Geometry: final body of the model. Coordinates: model frame, mm. Face numbers are marked on the shaded views. Coordinates: 2 decimals unless noted, no trailing zeros. Order: outer loops, then holes, each group sorted by start corner. A loop starts at its lowest first (then second) coordinate and runs counter-clockwise, first axis right, second up. Notation, with made-up numbers: M 65,31 L 116,31 A28 cw 116,51 Z; hole C 77,85 d1. An arc over 180 degrees is marked long. Write item = value, one per line.
from build123d import *

# Parameters (mm, degrees)
SALIENTE_EXTRUIR1_DEPTH = 0.5
CORTAR_EXTRUIR4_REACH   = 2.5
CROQUIS6_R              = 1.585
CORTAR_EXTRUIR5_REACH   = 2.5
CROQUIS7_R              = 1.585
CROQUIS8_R              = 1.585
CORTAR_EXTRUIR6_DEPTH   = 0.5
CROQUIS9_R              = 1.585
CORTAR_EXTRUIR7_DEPTH   = 0.5
CROQUIS5_R              = 1.585
CORTAR_EXTRUIR8_DEPTH   = 0.5
CORTAR_EXTRUIR9_REACH   = 182
CORTAR_EXTRUIR10_START  = -110.74
CORTAR_EXTRUIR10_DEPTH  = 110.74


with BuildPart() as part:
    # Croquis2 → Saliente-Extruir1 (new body)
    with BuildSketch(Plane(origin=(0, 0, 0), x_dir=(1, 0, 0), z_dir=(0, 1, 0))):
        Polygon((-90, 25.54), (-62.5, 25.54), (-62.5, 89.31), (62.5, 89.31), (62.5, 25.54), (90, 25.54), (90, -85.2), (-90, -85.2), align=None)
    saliente_extruir1 = extrude(amount=SALIENTE_EXTRUIR1_DEPTH)

    # Croquis6 → Cortar-Extruir4 (cut, up to next)
    with BuildSketch(Plane(origin=(0, 0.5, 0), x_dir=(1, 0, 0), z_dir=(0, 1, 0)), mode=Mode.PRIVATE) as cortar_extruir4_sk1:
        with Locations((-56.5, 35.81)):
            Circle(CROQUIS6_R)
    cortar_extruir4_tool1 = extrude(cortar_extruir4_sk1.sketch, amount=-CORTAR_EXTRUIR4_REACH, mode=Mode.PRIVATE) & part.part
    add(cortar_extruir4_tool1.solids().sort_by_distance((-56.5, 0.5, -35.81))[0], mode=Mode.SUBTRACT)
    # Croquis6 → Cortar-Extruir4 (cut, up to next)
    with BuildSketch(Plane(origin=(0, 0.5, 0), x_dir=(1, 0, 0), z_dir=(0, 1, 0)), mode=Mode.PRIVATE) as cortar_extruir4_sk2:
        with Locations((-15.5, 35.81)):
            Circle(CROQUIS6_R)
    cortar_extruir4_tool2 = extrude(cortar_extruir4_sk2.sketch, amount=-CORTAR_EXTRUIR4_REACH, mode=Mode.PRIVATE) & part.part
    add(cortar_extruir4_tool2.solids().sort_by_distance((-15.5, 0.5, -35.81))[0], mode=Mode.SUBTRACT)
    # Croquis6 → Cortar-Extruir4 (cut, up to next)
    with BuildSketch(Plane(origin=(0, 0.5, 0), x_dir=(1, 0, 0), z_dir=(0, 1, 0)), mode=Mode.PRIVATE) as cortar_extruir4_sk3:
        with Locations((-15.5, 84.31)):
            Circle(CROQUIS6_R)
    cortar_extruir4_tool3 = extrude(cortar_extruir4_sk3.sketch, amount=-CORTAR_EXTRUIR4_REACH, mode=Mode.PRIVATE) & part.part
    add(cortar_extruir4_tool3.solids().sort_by_distance((-15.5, 0.5, -84.31))[0], mode=Mode.SUBTRACT)
    # Croquis6 → Cortar-Extruir4 (cut, up to next)
    with BuildSketch(Plane(origin=(0, 0.5, 0), x_dir=(1, 0, 0), z_dir=(0, 1, 0)), mode=Mode.PRIVATE) as cortar_extruir4_sk4:
        with Locations((-56.5, 84.31)):
            Circle(CROQUIS6_R)
    cortar_extruir4_tool4 = extrude(cortar_extruir4_sk4.sketch, amount=-CORTAR_EXTRUIR4_REACH, mode=Mode.PRIVATE) & part.part
    add(cortar_extruir4_tool4.solids().sort_by_distance((-56.5, 0.5, -84.31))[0], mode=Mode.SUBTRACT)

    # Croquis7 → Cortar-Extruir5 (cut, up to next)
    with BuildSketch(Plane(origin=(0, 0.5, 0), x_dir=(1, 0, 0), z_dir=(0, 1, 0)), mode=Mode.PRIVATE) as cortar_extruir5_sk1:
        with Locations((56.5, 35.81)):
            Circle(CROQUIS7_R)
    cortar_extruir5_tool1 = extrude(cortar_extruir5_sk1.sketch, amount=-CORTAR_EXTRUIR5_REACH, mode=Mode.PRIVATE) & part.part
    add(cortar_extruir5_tool1.solids().sort_by_distance((56.5, 0.5, -35.81))[0], mode=Mode.SUBTRACT)
    # Croquis7 → Cortar-Extruir5 (cut, up to next)
    with BuildSketch(Plane(origin=(0, 0.5, 0), x_dir=(1, 0, 0), z_dir=(0, 1, 0)), mode=Mode.PRIVATE) as cortar_extruir5_sk2:
        with Locations((15.5, 35.81)):
            Circle(CROQUIS7_R)
    cortar_extruir5_tool2 = extrude(cortar_extruir5_sk2.sketch, amount=-CORTAR_EXTRUIR5_REACH, mode=Mode.PRIVATE) & part.part
    add(cortar_extruir5_tool2.solids().sort_by_distance((15.5, 0.5, -35.81))[0], mode=Mode.SUBTRACT)
    # Croquis7 → Cortar-Extruir5 (cut, up to next)
    with BuildSketch(Plane(origin=(0, 0.5, 0), x_dir=(1, 0, 0), z_dir=(0, 1, 0)), mode=Mode.PRIVATE) as cortar_extruir5_sk3:
        with Locations((15.5, 84.31)):
            Circle(CROQUIS7_R)
    cortar_extruir5_tool3 = extrude(cortar_extruir5_sk3.sketch, amount=-CORTAR_EXTRUIR5_REACH, mode=Mode.PRIVATE) & part.part
    add(cortar_extruir5_tool3.solids().sort_by_distance((15.5, 0.5, -84.31))[0], mode=Mode.SUBTRACT)
    # Croquis7 → Cortar-Extruir5 (cut, up to next)
    with BuildSketch(Plane(origin=(0, 0.5, 0), x_dir=(1, 0, 0), z_dir=(0, 1, 0)), mode=Mode.PRIVATE) as cortar_extruir5_sk4:
        with Locations((56.5, 84.31)):
            Circle(CROQUIS7_R)
    cortar_extruir5_tool4 = extrude(cortar_extruir5_sk4.sketch, amount=-CORTAR_EXTRUIR5_REACH, mode=Mode.PRIVATE) & part.part
    add(cortar_extruir5_tool4.solids().sort_by_distance((56.5, 0.5, -84.31))[0], mode=Mode.SUBTRACT)

    # Simetría3: Saliente-Extruir1 across plane
    add(saliente_extruir1.mirror(Plane(origin=(0, 0, 0), x_dir=(0, 0, 1), z_dir=(1, 0, 0))))

    # Croquis8 → Cortar-Extruir6 (cut)
    with BuildSketch(Plane(origin=(0, 0.5, 0), x_dir=(1, 0, 0), z_dir=(0, 1, 0))):
        with Locations((-20, 54.31)):
            Circle(CROQUIS8_R)
        with Locations((-47.5, 54.31)):
            Circle(CROQUIS8_R)
        with Locations((-47.5, 84.31)):
            Circle(CROQUIS8_R)
        with Locations((-20, 84.31)):
            Circle(CROQUIS8_R)
    cortar_extruir6 = extrude(amount=-CORTAR_EXTRUIR6_DEPTH, mode=Mode.SUBTRACT)

    # Simetría4: Cortar-Extruir6 across plane
    add(cortar_extruir6.mirror(Plane(origin=(0, 0, 0), x_dir=(0, 0, 1), z_dir=(1, 0, 0))), mode=Mode.SUBTRACT)

    # Croquis9 → Cortar-Extruir7 (cut)
    with BuildSketch(Plane.XZ):
        with Locations((56.5, -35.81)):
            Circle(CROQUIS9_R)
        with Locations((15.5, -35.81)):
            Circle(CROQUIS9_R)
        with Locations((15.5, -84.31)):
            Circle(CROQUIS9_R)
        with Locations((56.5, -84.31)):
            Circle(CROQUIS9_R)
    cortar_extruir7 = extrude(amount=-CORTAR_EXTRUIR7_DEPTH, mode=Mode.SUBTRACT)

    # Simetría5: Cortar-Extruir7 across plane
    add(cortar_extruir7.mirror(Plane(origin=(0, 0, 0), x_dir=(0, 0, 1), z_dir=(1, 0, 0))), mode=Mode.SUBTRACT)

    # Croquis5 → Cortar-Extruir8 (cut)
    with BuildSketch(Plane(origin=(0, 0.5, 0), x_dir=(1, 0, 0), z_dir=(0, 1, 0))):
        with Locations((74, -24.969940997)):
            Circle(CROQUIS5_R)
    cortar_extruir8 = extrude(amount=-CORTAR_EXTRUIR8_DEPTH, mode=Mode.SUBTRACT)

    # Simetría6: Cortar-Extruir8 across plane
    add(cortar_extruir8.mirror(Plane(origin=(0, 0, 0), x_dir=(0, 0, 1), z_dir=(1, 0, 0))), mode=Mode.SUBTRACT)

    # Croquis3 → Cortar-Extruir9 (cut, up to next)
    with BuildSketch(Plane(origin=(90, 0, 0), x_dir=(0, 0, -1), z_dir=(1, 0, 0)), mode=Mode.PRIVATE) as cortar_extruir9_sk1:
        Polygon((-85.2, 0), (-83.82626129, 0.5), (-85.2, 0.5), align=None)
    cortar_extruir9_tool1 = extrude(cortar_extruir9_sk1.sketch, amount=-CORTAR_EXTRUIR9_REACH, mode=Mode.PRIVATE) & part.part
    add(cortar_extruir9_tool1.solids().sort_by_distance((90, 0.333333, 84.742087))[0], mode=Mode.SUBTRACT)

    # Croquis10 → Cortar-Extruir10 (cut)
    with BuildSketch(Plane(origin=(0, 0, -25.54), x_dir=(-1, 0, 0), z_dir=(0, 0, -1)).offset(CORTAR_EXTRUIR10_START)):
        Polygon((90, 0), (90, 0.5), (88.62626129, 0.5), align=None)
    cortar_extruir10 = extrude(amount=CORTAR_EXTRUIR10_DEPTH, mode=Mode.SUBTRACT)

    # Simetría7: Cortar-Extruir10 across plane
    add(cortar_extruir10.mirror(Plane(origin=(0, 0, 0), x_dir=(0, 0, 1), z_dir=(1, 0, 0))), mode=Mode.SUBTRACT)


solid = part.part
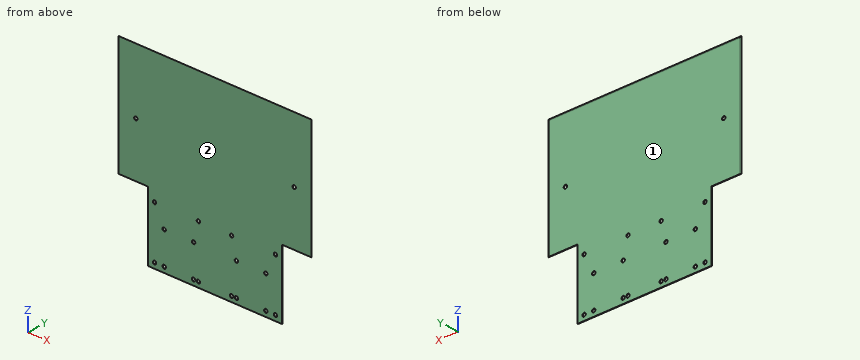
1) Section B-B, the plane z = -66.5. Return loops of the section in (x, y), and give its area (3 significant figures).
Numbers:
outline = M -62.5,0 L 62.5,0 L 62.5,0.5 L -62.5,0.5 Z
area = 62.5 mm²
2) Section A-A, the plane y = 0.1. Give the number of separate pieces and of enclosed holes in the cut face, and give its area (3 significant figures).
Numbers:
separate_pieces = 1
enclosed_holes = 18
area = 27,700 mm²
3) Mould query, pull axis Y, two halves, no side actions, for the marked faces 1 and 2. Classes: pulls with the +Y half, pulls with the -Y half, needs draft (parallel to the pull), parting line crosses it, or undercut.
Numbers:
face_1 = pulls with the +Y half
face_2 = pulls with the -Y half
